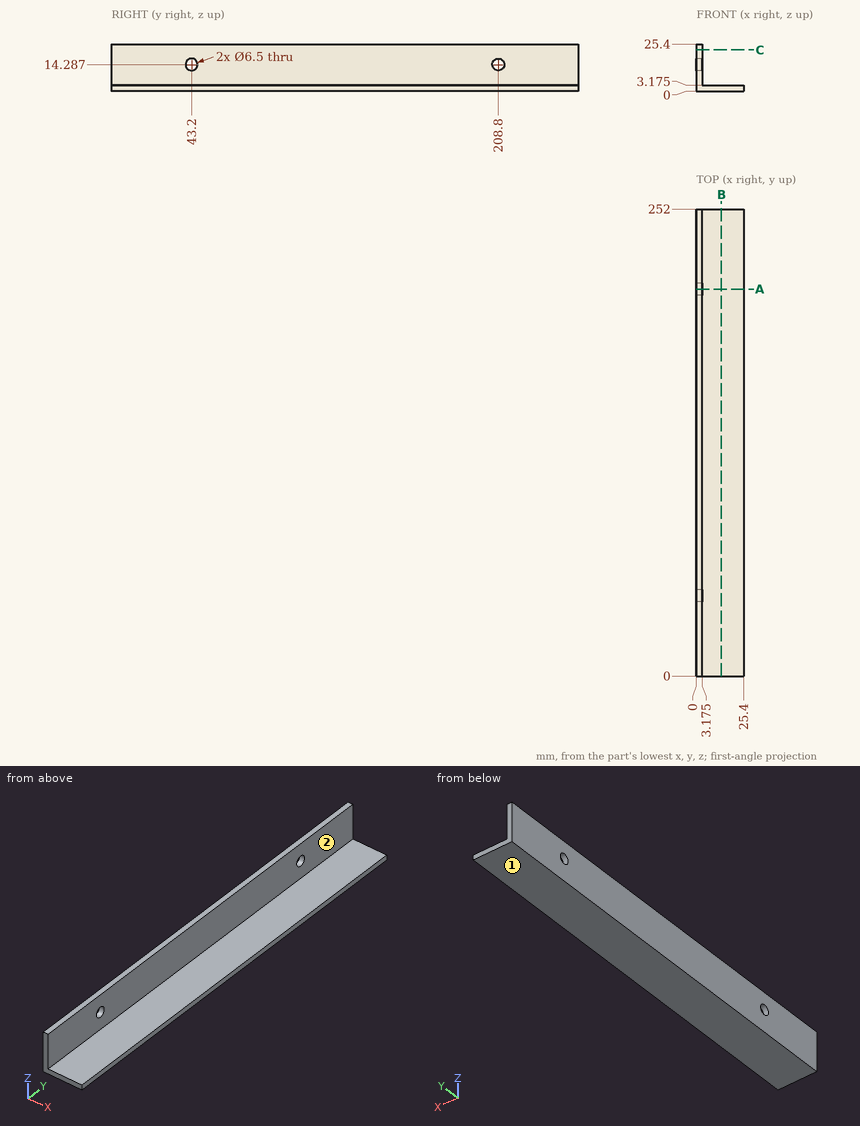
Design review of the part shown in the three views and the two pictorial views. Dimensions are in mm from the part's minimum x, y and z. A direction names the side the tool comes from. Round coordinates to 2 decimals unless told otherwise and drop trailing zeros. Write each loop counter-clockwise with the first axis right and the second up, starting at its lowest first coordinate (ties: lowest second). Pieces come first, ordered by that corner, then holes.
1) Take a section at A-A on y = 208.8. Give the boundary of the cut face in (x, z) (1 decimal).
Answer below:
outline: (0, 0) - (25.4, 0) - (25.4, 3.2) - (3.2, 3.2) - (3.2, 11) - (0, 11) - close; (0, 17.5) - (3.2, 17.5) - (3.2, 25.4) - (0, 25.4) - close
2) Insertion check: pin 1 Ø12 at (x, y) = (19, 82) entering from +Z (1 decimal); pin 2 Ø11 at (y, z) = (184.5, 16.5) entering from +X (1 decimal); pin 3 Ø10 at (x, z) = (10.5, 14.5) entering from +Y. Each pin has a flat end and moves straight along its axis. Give the tip position at first contact, or say it passes through.
Answer below:
pin 1: stops at z = 3.2
pin 2: stops at x = 3.2
pin 3: passes through
3) For line 1 along Z through (x, y) = (1.95, 208.8); line 2 along X through (y, z) = (35, 13.5) (1 decimal), list the stretches that pass through material, from the lowest coordinate up.
Answer below:
line 1: z = 0 to 11.04, 17.54 to 25.4
line 2: x = 0 to 3.2
4) Take a section at B-B on x = 13.5. Give the boundary of the cut face in (y, z) (1 decimal).
Answer below:
outline: (0, 0) - (252, 0) - (252, 3.2) - (0, 3.2) - close
5) Machinability: for the marked faces 1 and 2, which of the approach directions +Z, -Z, +X, -X, +Y, -Y give a long, thin tool a straight path to every point of the face, cutting with its end or side? Answer none if there is none.
Answer below:
face 1: -Z, +X, -X, +Y, -Y
face 2: +Z, +X, +Y, -Y
6) Take a section at C-C on z = 22.25. Give the boundary of the cut face in (x, y) (1 decimal).
Answer below:
outline: (0, 0) - (3.2, 0) - (3.2, 252) - (0, 252) - close
